Autodesk Inventor part; units mm, degrees
ref_plane "YZ Plane" through (0, 0, 0) normal (1, 0, 0) x (0, 1, 0)
ref_plane "XZ Plane" through (0, 0, 0) normal (0, 1, 0) x (-1, 0, 0)
ref_plane "XY Plane" through (0, 0, 0) normal (0, 0, 1) x (1, 0, 0)
sketch "Sketch14" plane through (0, 0, 0) normal (0, 0, 1) x (1, 0, 0)
  line L0 (0, 0) -> (17, 0)
  line L1 (17, 0) -> (17, 30)
  line L2 (17, 30) -> (0, 30)
  line L3 (0, 30) -> (0, 0)
  line L4 (-6, 36) -> (23, 36)
  line L5 (23, 36) -> (23, -6)
  line L6 (23, -6) -> (-6, -6)
  line L7 (-6, -6) -> (-6, 36)
  dimension "d55" = 17
  dimension "d56" = 30
  dimension "d57" = 6
extrude "Extrusion12" add sketch "Sketch14" against normal blind 3 contours L3 L2 L1 L0 | L4 L5 L6 L7
extrude "Extrusion13" add sketch "Sketch14" along normal blind 90 contours L3 L2 L1 L0
sketch "Sketch15" plane through (0, 0, 0) normal (0, -1, 0) x (1, 0, 0)
  line L0 (0, 0) -> (0, 90)
  line L1 (0, 90) -> (17.1111, 90)
  line L2 (0, 90) -> (17, 90)
  line L3 (17, 90) -> (17, 97)
  line L4 (17, 97) -> (0, 97)
  line L5 (0, 97) -> (0, 90)
  line L6 (17, 90) -> (0, 90)
  circle A0 centre (8.5, 78.8) radius 7.15
  line L7 (17, 0) -> (17, 90)
  line L8 (0, 97) -> (17, 97)
  line L9 (17, 97) -> (17, 42)
  line L10 (17, 42) -> (0, 42)
  line L11 (0, 42) -> (0, 97)
  dimension "d67" = 7
  dimension "d73" = 14.3
  dimension "d79" = 55
extrude "Extrusion14" cut sketch "Sketch15" against normal blind 90 contours A0
extrude "Extrusion15" cut sketch "Sketch15" against normal blind 15.5 contours L0 L1 L7 L10
extrude "Extrusion17" add sketch "Sketch15" against normal blind 30 contours L5 L4 L3 L1
sketch "Sketch16" plane through (0, 0, 0) normal (0, -1, 0) x (1, 0, 0)
  line L0 (0, 0) -> (0, 97)
  line L1 (17, 0) -> (17, 97)
  line L2 (0, 97) -> (17, 97)
  line L3 (17, 97) -> (17, 90)
  line L4 (17, 90) -> (0, 90)
  line L5 (0, 90) -> (0, 97)
  dimension "d86" = 7
extrude "Extrusion18" cut sketch "Sketch15" against normal blind 15.5 contours L5 L4 L3 L1
sketch "Sketch21" plane through (0, 15.5, 97) normal (0, 0, 1) x (1, 0, 0)
  line L0 (0, 14.5) -> (17, 14.5)
  line L1 (0, 14.5) -> (0, 16.5)
  line L2 (0, 16.5) -> (-2, 16.5)
  line L3 (17, 0) -> (19, 0)
  line L4 (19, 0) -> (19, -2)
  line L5 (-2, 16.5) -> (19, 16.5)
  line L6 (19, 16.5) -> (19, -2)
  line L7 (19, -2) -> (-2, -2)
  line L8 (-2, -2) -> (-2, 16.5)
  point P0 (0, -15.5)
  dimension "d109" = 2
  dimension "d110" = 2
  dimension "d111" = 2
  dimension "d112" = 2
extrude "Extrusion24" add sketch "Sketch21" against normal blind 97.9375
sketch "Sketch22" plane through (0, 0, 42) normal (0, 0, 1) x (1, 0, 0)
  line L0 (17, 13.5) -> (0, 13.5)
  line L1 (0, 13.5) -> (17.0001, 13.5)
  line L2 (17.0001, 13.5) -> (17.0001, 0)
  line L3 (17.0001, 0) -> (0, 0)
  line L4 (0, 0) -> (0, 13.5)
extrude "Extrusion25" cut sketch "Sketch22" against normal blind 42
extrude "Extrusion26" cut sketch "Sketch15" against normal blind 97.9375 contours A0
sketch "Sketch23" plane through (0, 0, -3) normal (0, 0, -1) x (-1, 0, 0)
  line L0 (-28.2805, -15.4048) -> (9.4268, -15.4048)
  line L1 (9.4268, -15.4048) -> (9.4268, 47.594)
  line L2 (9.4268, 47.594) -> (-28.2805, 47.594)
  line L3 (-28.2805, 47.594) -> (-28.2805, -15.4048)
  point P0 (0, 0)
extrude "Extrusion27" cut sketch "Sketch23" against normal blind 43
sketch "Sketch24" plane through (-2, 32, 97) normal (0, 1, 0) x (1, 0, 0)
  point P0 (2, 97)
sketch "Sketch25" plane through (-2, 32, 97) normal (0, 1, 0) x (1, 0, 0)
  point P0 (2, 97)
sketch "Sketch26" plane through (-2, 32, 97) normal (0, 1, 0) x (1, 0, 0)
  point P0 (2, 97)
sketch "Sketch27" plane through (-2, 32, 97) normal (0, 1, 0) x (1, 0, 0)
  point P0 (2, 97)
sketch "Sketch28" plane through (-2, 32, 97) normal (0, 1, 0) x (1, 0, 0)
  point P0 (2, 97)
sketch "Sketch29" plane through (-2, 32, 97) normal (0, 1, 0) x (1, 0, 0)
  point P0 (2, 97)
sketch "Sketch30" plane through (-2, 32, 97) normal (0, 1, 0) x (1, 0, 0)
  point P0 (2, 97)
  point P1 (21, 0)
  point P2 (0, 57)
sketch "Sketch31" plane through (0, 0, 40) normal (0, 0, -1) x (-1, 0, 0)
  line L0 (2, 13.5) -> (-19, 13.5)
  line L1 (-19, 32) -> (2, 32)
  line L2 (2, 13.5) -> (-19, 13.5)
  line L3 (-19, 13.5) -> (-19, 32)
  line L4 (-19, 32) -> (2, 32)
  line L5 (2, 32) -> (2, 13.5)
  point P0 (0, 0)
  point P1 (2, 32)
extrude "Extrusion28" add sketch "Sketch31" along normal blind 43
sketch "Sketch33" plane through (-2, 13.5, 97) normal (0, 0, 1) x (1, 0, 0)
  line L0 (0, 0) -> (21, 0)
  line L1 (0, 0) -> (-2, 0)
  line L2 (-2, 0) -> (-2, 18.5)
  line L3 (-2, 18.5) -> (0, 18.5)
  line L4 (0, 18.5) -> (0, 0)
  line L5 (21, 0) -> (21, 18.5)
  line L6 (21, 0) -> (23, 0)
  line L7 (23, 0) -> (23, 18.5)
  line L8 (23, 18.5) -> (21, 18.5)
  line L9 (21, 18.5) -> (21, 0)
  point P0 (2, -13.5)
  dimension "d123" = 2
  dimension "d124" = 2
extrude "Extrusion29" add sketch "Sketch33" against normal blind 100
sketch "Sketch37" plane through (0, 0, -3) normal (0, 0, -1) x (-1, 0, 0)
  line L0 (-21, 32) -> (-21, 13.5)
  line L1 (4, 13.5) -> (-21, 13.5)
  line L2 (-21, 32) -> (4, 32)
  line L3 (4, 32) -> (4, 13.5)
  line L4 (4, 13.5) -> (-21, 13.5)
  line L5 (-21, 13.5) -> (-21, 32)
  point P0 (0, 0)
extrude "Extrusion30" add sketch "Sketch37" along normal blind 17
sketch "Sketch38" plane through (0, 0, -20) normal (0, 0, -1) x (-1, 0, 0)
  line L0 (4, 13.5) -> (-21, 13.5)
  line L1 (4, 13.5) -> (10.5, 13.5)
  line L2 (10.5, 13.5) -> (10.5, 32)
  line L3 (10.5, 32) -> (4, 32)
  line L4 (4, 32) -> (4, 13.5)
  line L5 (-21, 13.5) -> (-21, 32)
  line L6 (-21, 13.5) -> (-27.5, 13.5)
  line L7 (-27.5, 13.5) -> (-27.5, 32)
  line L8 (-27.5, 32) -> (-21, 32)
  line L9 (-21, 32) -> (-21, 13.5)
  line L10 (-27.5, 32) -> (10.5, 32)
  line L11 (10.5, 32) -> (10.5, 36)
  line L12 (10.5, 36) -> (-27.5, 36)
  line L13 (-27.5, 36) -> (-27.5, 32)
  line L14 (-24.25, 13.5) -> (-24.25, 18)
  line L15 (-24.25, 36) -> (-24.25, 30.5)
  line L16 (7.25, 36) -> (7.25, 30.5)
  line L17 (7.25, 13.5) -> (7.25, 18)
  circle A0 centre (-24.25, 30.5) radius 1.5
  circle A1 centre (-24.25, 18) radius 1.5
  circle A2 centre (7.25, 18) radius 1.5
  circle A3 centre (7.25, 30.5) radius 1.5
  line L18 (-24.25, 31.5) -> (-24.25, 30.5)
  line L19 (7.25, 31.5) -> (7.25, 30.5)
  line L20 (-27.5, 36) -> (10.5, 36)
  line L21 (10.5, 36) -> (10.5, 35)
  line L22 (10.5, 35) -> (-27.5, 35)
  line L23 (-27.5, 35) -> (-27.5, 36)
  line L24 (7.25, 35) -> (10.5, 35)
  line L25 (10.5, 35) -> (10.5, 32)
  line L26 (10.5, 32) -> (7.25, 32)
  line L27 (7.25, 32) -> (7.25, 35)
  point P0 (0, 0)
  point P1 (7.25, 32)
  point P2 (7.25, 32)
  point P3 (7.25, 32)
  point P4 (7.25, 35)
  dimension "d132" = 4.5
  dimension "d135" = 4.5
  dimension "d137" = 3
  dimension "d138" = 3
  dimension "d142" = 1
  dimension "d143" = 1
extrude "Extrusion31" add sketch "Sketch38" along normal blind 4 contours L4 L3 L2 L1 | L0 L5 L10 L4 | L6 L7 L8 L5 | L10 L8 L15 L22 L16 L3 | L16 L22 L11 L3 | L8 L13 L22 L15
properties part number "ramie_2"
Model file for the job. Use its own axes, mm. A direction names the side the tool comes from. Give positions to 0.01 mm unless a question says otherwise; leave off trailing zeros. Order: outer loops, then holes, each group sorted by start corner. A loop starts at its lowest first (then second) coordinate and runs counter-clockwise, first axis right, second up. Notation, with made-up numbers: M 12.25,35.5 L 21.25,35.5 A19 ccw 21.25,63.5 Z; hole C 15.5,6 d1. An arc over 180 degrees is marked long. Put each result on its own line as item: value. Start each with the question number.
(1) Pull direction Z, two halves, no side cores. Call faces 4 (the face through (6.95, 22.62, 71.82)), 5 (the face through (9, 24, -24)), 6 (the face through (8, 23, 97)): released by +Z, released by -Z, zero draft, split by the parting line, or undercut.
(2) Tool access for faces 1 (the face through (21, 23, 39)), 2 (the face through (-4, 23, 39)), 3 (the face through (9, 32, 39)): list every direction of +Z, -Z, +X, -X, +Y, -Y with a clear straight run to the whole face (end or side of a thin tool).
(3) Drill centre lines: L1, parallel to Y at x = -7.25, z = -22.4; L2, parallel to X at y = 18, z = -22.7; L3, parallel to Z at x = 9, y = 22.5. Where is each one in solid material? Low to high. Write a range as [from, to].
(4) Band-saw the part on A-A on y = 18. Give the cut face in (x, z), then the cut area to 3 significant figures.
(5) Band-saw the part on C-C on x = 8.5. Give the cut face in (y, z), then the cut area to 3 significant figures.
(6) Band-saw the part on D-D on z = 6. Give the cut face in (x, y).
(7) Band-saw the part on B-B on x = 24.25. Give the cut face in (y, z).
(8) Pin check, flat tips, straight feed: pin 1 Ø2.5 at (x, y) = (24.25, 18) entering from +Z; pin 2 Ø8 at (x, z) = (16, 60.5) entering from +Y; pin 3 Ø1.5 at (y, z) = (30.5, -3) entering from +X; pin 4 Ø3.5 at (x, y) = (-7.25, 18) entering from -Z. Stop position of each tip, or through.
Results below:
1. face 4: undercut
1. face 5: released by -Z
1. face 6: released by +Z
2. face 1: +Z, +X, +Y, -Y
2. face 2: +Z, -X, +Y, -Y
2. face 3: +Z, +X, -X, +Y
3. L1: y = [13.5, 16.5], [19.5, 29], [32, 35]
3. L2: x = [-10.5, -8.75], [-5.75, 22.75], [25.75, 27.5]
3. L3: z = [-24, 71.67], [85.93, 97]
4. outline: M -10.5,-24 L -8.75,-24 L -8.75,-20 L -10.5,-20 Z; M -5.75,-24 L 22.75,-24 L 22.75,-20 L 21,-20 L 21,97 L -4,97 L -4,-20 L -5.75,-20 Z; M 25.75,-24 L 27.5,-24 L 27.5,-20 L 25.75,-20 Z; hole C 8.5,78.8 d14.3
4. area: 2,890 mm2
5. outline: M 13.5,-24 L 35,-24 L 35,-20 L 32,-20 L 32,71.65 L 13.5,71.65 Z; M 13.5,85.95 L 32,85.95 L 32,97 L 13.5,97 Z
5. area: 1,990 mm2
6. outline: M -4,13.5 L 21,13.5 L 21,32 L -4,32 Z
7. outline: M 13.5,-24 L 16.5,-24 L 16.5,-20 L 13.5,-20 Z; M 19.5,-24 L 29,-24 L 29,-20 L 19.5,-20 Z; M 32,-24 L 35,-24 L 35,-20 L 32,-20 Z
8. pin 1: passes through
8. pin 2: stops at y = 32
8. pin 3: stops at x = 21
8. pin 4: stops at z = -24
